Source: CAD feature listing. Evaluate the final solid. Frame: model axes, mm. Face numbers are marked on the shaded views. Coordinates: 2 decimals unless noted, no trailing zeros. Loops run counter-clockwise (first coordinate to the right, second up) from the corner with the lowest first, then second, coordinate; pieces in that order, holes last. Notation, with made-up numbers: (-9, 6) -> (3, 6) arc R28 cw to (3, 33) -> close; hole circle Ø1 at (-23.5, -4). An arc over 180 degrees is marked (long way). Answer as CSV lines item,"result".
from build123d import *

# Parameters (mm, degrees)
SKETCH014_W          = 25
SKETCH014_H          = 25
SKETCH014_R          = 3
PAD007_DEPTH         = 12.5
SKETCH015_R          = 3.4
POCKET007_DEPTH      = 12.501
POCKET007_DEPTH_BACK = 12.501
CHAMFER001_SIZE      = 1
SKETCH020_R          = 2.5
POCKET009_DEPTH      = 12.501
POCKET009_DEPTH_BACK = 12.501


with BuildPart() as part:
    # Sketch014 → Pad007 (new body, symmetric)
    with BuildSketch(Plane.YZ):
        Rectangle(SKETCH014_W, SKETCH014_H)
        with Locations((1.5, 1)):
            Circle(SKETCH014_R, mode=Mode.SUBTRACT)
    extrude(amount=PAD007_DEPTH, both=True)

    # Sketch015 → Pocket007 (cut, two sides)
    with BuildSketch(Plane.XZ) as pocket007_sk:
        with Locations((0, -6.9)):
            Circle(SKETCH015_R)
    extrude(amount=-POCKET007_DEPTH, mode=Mode.SUBTRACT)
    extrude(pocket007_sk.sketch, amount=POCKET007_DEPTH_BACK, mode=Mode.SUBTRACT)

    # Chamfer001
    chamfer001_edges = [part.edges().sort_by_distance(p)[0] for p in [
        (-12.5, 0, 12.5),
        (-12.5, 12.5, 0),
        (-12.5, 0, -12.5),
        (-12.5, -12.5, 0),
        (-12.5, -1.5, 1),
        (12.5, 0, 12.5),
        (12.5, 12.5, 0),
        (12.5, 0, -12.5),
        (12.5, -12.5, 0),
        (12.5, -1.5, 1),
        (0, -12.5, 12.5),
        (0, 12.5, 12.5),
        (0, 12.5, -12.5),
        (0, -12.5, -12.5),
    ]]
    chamfer(chamfer001_edges, length=CHAMFER001_SIZE)

    # Sketch020 → Pocket009 (cut, two sides)
    with BuildSketch(Plane.XZ) as pocket009_sk:
        with Locations((0, 7.5)):
            Circle(SKETCH020_R)
    extrude(amount=-POCKET009_DEPTH, mode=Mode.SUBTRACT)
    extrude(pocket009_sk.sketch, amount=POCKET009_DEPTH_BACK, mode=Mode.SUBTRACT)


with BuildPart() as part_1:
    # Body005 placement: moved
    add(part.part.moved(Location((0, -36.5, -10.5))))


solid = part_1.part
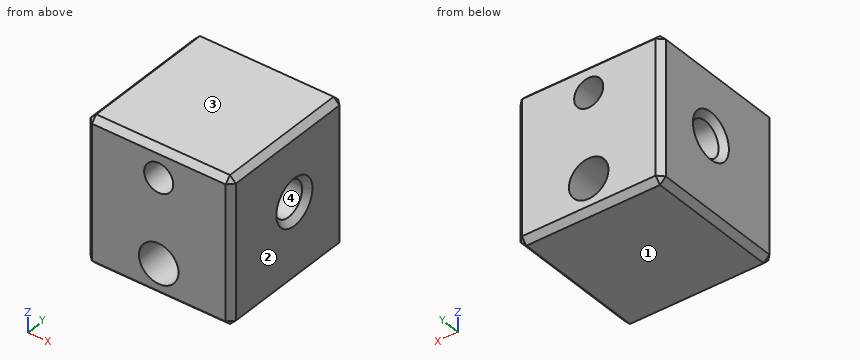
(1) Material intervals for L1, parallel to Z at x = 0, y = -39.5; L2, parallel to Z at x = 1, y = -27; L3, parallel to X at y = -39.75, z = -17.4, sorted ascending. Write a range as [from, to].
Computed values:
L1,"[-23, -20.8], [-14, -5.5], [-0.5, 2]"
L2,"[-23, -20.65], [-14.15, -5.29], [-0.71, 2]"
L3,"[-12.5, -3.4], [3.4, 12.5]"
(2) Pin query (flat end, axial travel): pin 1 Ø4 at (x, z) = (0, -3) entering from -Y; pin 2 Ø7 at (y, z) = (-35, -9.5) entering from +X. Return the tip coordinate at first contact, or that it passes through.
Computed values:
pin 1,"through"
pin 2,"x = 12"
(3) Cut plane A-A (z = -5). Return the cut outline in (x, y).
Computed values:
outline,"(-12.5, -48) -> (-11.5, -49) -> (-1.5, -49) -> (-1.5, -24) -> (-11.5, -24) -> (-12.5, -25) -> close; (1.5, -49) -> (11.5, -49) -> (12.5, -48) -> (12.5, -25) -> (11.5, -24) -> (1.5, -24) -> close"
(4) Cut plane B-B (y = -35). Return the cut outline in (x, z), then the cut area to 3 significant figures.
Computed values:
outline,"(-12.5, -22) -> (-11.5, -23) -> (11.5, -23) -> (12.5, -22) -> (12.5, -13.5) -> (11.5, -12.5) -> (-11.5, -12.5) -> (-12.5, -13.5) -> close; (-12.5, -5.5) -> (-11.5, -6.5) -> (11.5, -6.5) -> (12.5, -5.5) -> (12.5, 1) -> (11.5, 2) -> (-11.5, 2) -> (-12.5, 1) -> close; hole circle Ø6.8 at (0, -17.4); hole circle Ø5 at (0, -3)"
area,"415 mm^2"
(5) Draft query along Z for the marked faces 1, 2, 3 and 4. Return one class per face: released by +Z, released by -Z, zero draft, split by the parting line, or undercut.
Computed values:
face 1,"released by -Z"
face 2,"zero draft"
face 3,"released by +Z"
face 4,"undercut"
(6) Cut plane C-C (x = 0). Return the cut outline in (y, z).
Computed values:
outline,"(-49, -22) -> (-48, -23) -> (-25, -23) -> (-24, -22) -> (-24, -20.8) -> (-49, -20.8) -> close; (-49, -14) -> (-24, -14) -> (-24, -5.5) -> (-49, -5.5) -> close; (-49, -0.5) -> (-24, -0.5) -> (-24, 1) -> (-25, 2) -> (-48, 2) -> (-49, 1) -> close; hole circle Ø6 at (-35, -9.5)"
(7) Cut plane D-D (x = 4). Return the cut outline in (y, z).
Computed values:
outline,"(-49, -22) -> (-48, -23) -> (-25, -23) -> (-24, -22) -> (-24, 1) -> (-25, 2) -> (-48, 2) -> (-49, 1) -> close; hole circle Ø6 at (-35, -9.5)"
